Source: three-view drawing plus pictorial views. Frame: mm from the lowest corner of the part. A direction names the side the tool comes from. Give positions to 0.01 mm unless a question says otherwise; leave off trailing zeros. Loops run counter-clockwise (first coordinate to the right, second up) from the corner with the lowest first, then second, coordinate; pieces in that order, holes last. Notation, with made-up numbers: (21, -13) - (42, -13) arc R21 cw to (42, 19) - close; hole circle Ø5 at (63.25, 30.25). An arc over 180 degrees is marked (long way). Answer in a Markdown table with one row per item.
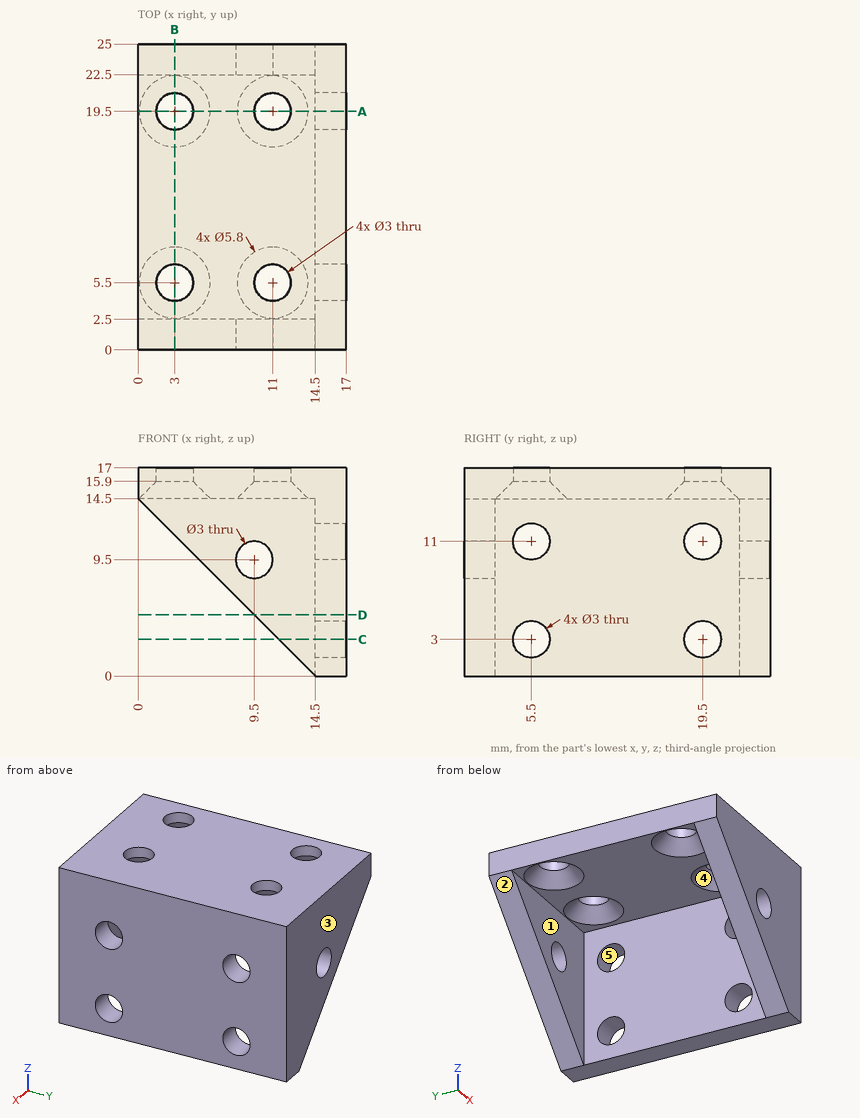
Q1. Cut plane D-D (z = 5). Output: boundary loops of the cut face in (x, y).
Check values:
| item | result |
|---|---|
| outline | (9.5, 0) - (17, 0) - (17, 25) - (9.5, 25) - (9.5, 22.5) - (14.5, 22.5) - (14.5, 2.5) - (9.5, 2.5) - close |
Q2. Cut plane B-B (x = 3). Output: boundary loops of the cut face in (y, z).
Check values:
| item | result |
|---|---|
| outline | (0, 11.5) - (2.5, 11.5) - (2.5, 14.5) - (2.6, 14.5) - (4, 15.9) - (4, 17) - (0, 17) - close; (7, 15.9) - (8.4, 14.5) - (16.6, 14.5) - (18, 15.9) - (18, 17) - (7, 17) - close; (21, 15.9) - (22.4, 14.5) - (22.5, 14.5) - (22.5, 11.5) - (25, 11.5) - (25, 17) - (21, 17) - close |
Q3. Cut plane C-C (z = 3). Output: boundary loops of the cut face in (x, y), and give its area (3 significant figures).
Check values:
| item | result |
|---|---|
| outline | (11.5, 0) - (17, 0) - (17, 4) - (14.5, 4) - (14.5, 2.5) - (11.5, 2.5) - close; (11.5, 22.5) - (14.5, 22.5) - (14.5, 21) - (17, 21) - (17, 25) - (11.5, 25) - close; (14.5, 7) - (17, 7) - (17, 18) - (14.5, 18) - close |
| area | 62.5 mm² |
Q4. Cut plane A-A (y = 19.5). Output: boundary loops of the cut face in (x, z), and give its area (3 significant figures).
Check values:
| item | result |
|---|---|
| outline | (0, 14.5) - (0.1, 14.5) - (1.5, 15.9) - (1.5, 17) - (0, 17) - close; (4.5, 15.9) - (5.9, 14.5) - (8.1, 14.5) - (9.5, 15.9) - (9.5, 17) - (4.5, 17) - close; (12.5, 15.9) - (13.9, 14.5) - (14.5, 14.5) - (14.5, 12.5) - (17, 12.5) - (17, 17) - (12.5, 17) - close; (14.5, 0) - (17, 0) - (17, 1.5) - (14.5, 1.5) - close; (14.5, 4.5) - (17, 4.5) - (17, 9.5) - (14.5, 9.5) - close |
| area | 44.8 mm² |
Q5. Reachability of the marked faces 1 and 2 from +Z, -Z, +X, -X, +Y, -Y: full face, straight path, thin tool, end or side. Return the list, or none.
Check values:
| item | result |
|---|---|
| face 1 | -Z, -X |
| face 2 | -Z, -X, +Y, -Y |
Q6. Material intervals for line 1 along Y through (x, z) = (3, 16.15); line 2 along X through (y, z) = (5.5, 16.6); line 3 along X through (y, z) = (4.25, 14.75), sorted ascending.
Check values:
| item | result |
|---|---|
| line 1 | 0 to 4, 7 to 18, 21 to 25 |
| line 2 | 0 to 1.5, 4.5 to 9.5, 12.5 to 17 |
| line 3 | 0 to 0.66, 5.34 to 8.66, 13.34 to 17 |
Q7. Draft query along Z for the marked faces 3, 4 and 5. Return one class per face: pulls with the +Z half, pulls with the -Z half, needs draft (parallel to the pull), parting line crosses it, or undercut.
Check values:
| item | result |
|---|---|
| face 3 | needs draft |
| face 4 | pulls with the -Z half |
| face 5 | undercut |
Q8. First-contact query: pin 1 (4 mm diameter, centred on y = 19, z = 6.5, fed in from -X); pin 2 (2.5 mm diameter, centred on y = 19.5, z = 3, fed in from -X); pin 3 (4 mm diameter, centred on x = 11.5, y = 16.5, fed in from -Z); pin 4 (5 mm diameter, centred on x = 3, y = 19.5, fed in from -Z). Flat tips, straight axial feed; report the tip coordinate or a pass-through.
Check values:
| item | result |
|---|---|
| pin 1 | x = 14.5 |
| pin 2 | through |
| pin 3 | z = 14.5 |
| pin 4 | z = 14.9 |
